```python
from build123d import *

# Parameters (mm, degrees)
F1_DEPTH  = 40
F3_DEPTH  = 15
F4_DEPTH  = 20
F6_DEPTH  = 15
F8_DEPTH  = 15
F9_R      = 7.5
F10_DEPTH = 70
F13_DEPTH = 6
F11_W     = 22
F11_H     = 56
F14_DEPTH = 6
F15_R     = 9.5
F16_DEPTH = 30
F15_R_2   = 19.5
F17_DEPTH = 12
F18_R     = 10


with BuildPart() as f1:
    # F0 (on Front) → F1 (new body, symmetric)
    with BuildSketch(Plane.XZ):
        Polygon((-30.7818128993, 84.5723358707), (0, 0), (130, 0), (130, 15), (115, 15), (45, 15), (10.5031130731, 15), (-11.5561214376, 75.6072487088), (22.2728129107, 87.9199738686), (17.1425107608, 102.0153631803), align=None)
    extrude(amount=F1_DEPTH, both=True)

    # F2 (on face) → F3 (join)
    with BuildSketch(Plane(origin=(-30.7818128993, 0, 84.5723358707), x_dir=(0.9396926208, 0, 0.3420201433), z_dir=(-0.3420201433, 0, 0.9396926208))):
        with BuildLine():
            Line((51, 40), (51, -40))
            ThreePointArc((51, -40), (91, 0), (51, 40))
        make_face()
    extrude(amount=-F3_DEPTH)

    # F0 (on Front) → F4 (join, symmetric)
    with BuildSketch(Plane.XZ):
        Polygon((-30.7818128993, 84.5723358707), (0, 0), (130, 0), (130, 15), (115, 15), (45, 15), (10.5031130731, 15), (-11.5561214376, 75.6072487088), (22.2728129107, 87.9199738686), (17.1425107608, 102.0153631803), align=None)
        Polygon((45, 15), (115, 15), (115, 55), (100, 55), (100, 22), (60, 22), (60, 55), (45, 55), align=None)
    extrude(amount=F4_DEPTH, both=True)

    # F5 (on face) → F6 (join)
    with BuildSketch(Plane.YZ.offset(115)):
        with BuildLine():
            Line((-20, 55), (20, 55))
            ThreePointArc((20, 55), (0, 75), (-20, 55))
        make_face()
    extrude(amount=-F6_DEPTH)

    # F7 (on face) → F8 (join)
    with BuildSketch(Plane.YZ.offset(60)):
        with BuildLine():
            Line((-20, 55), (20, 55))
            ThreePointArc((20, 55), (0, 75), (-20, 55))
        make_face()
    extrude(amount=-F8_DEPTH)

    # F9 (on face) → F10 (cut)
    with BuildSketch(Plane.YZ.offset(115)):
        with Locations((0, 55)):
            Circle(F9_R)
    extrude(amount=-F10_DEPTH, mode=Mode.SUBTRACT)

    # F12 (on face) → F13 (cut)
    with BuildSketch(Plane(origin=(-30.7818128993, 0, 84.5723358707), x_dir=(0.9396926208, 0, 0.3420201433), z_dir=(-0.3420201433, 0, 0.9396926208))):
        with BuildLine():
            Line((89.4577690461, 11), (0, 11))
            Line((0, 11), (0, -11))
            Line((0, -11), (89.4577690461, -11))
            ThreePointArc((89.4577690461, -11), (91, 0), (89.4577690461, 11))
        make_face()
    extrude(amount=-F13_DEPTH, mode=Mode.SUBTRACT)

    # F11 (on face) → F14 (cut)
    with BuildSketch(Plane(origin=(0, 0, 0), x_dir=(0, -1, 0), z_dir=(-0.9396926208, 0, -0.3420201433))):
        with Locations((0, 62)):
            Rectangle(F11_W, F11_H)
    extrude(amount=-F14_DEPTH, mode=Mode.SUBTRACT)

    # F15 (on face) → F16 (cut)
    with BuildSketch(Plane(origin=(-30.7818128993, 0, 84.5723358707), x_dir=(0.9396926208, 0, 0.3420201433), z_dir=(-0.3420201433, 0, 0.9396926208))):
        with Locations((51, 0)):
            Circle(F15_R)
    extrude(amount=-F16_DEPTH, mode=Mode.SUBTRACT)

    # F15 (on face) → F17 (cut)
    with BuildSketch(Plane(origin=(-30.7818128993, 0, 84.5723358707), x_dir=(0.9396926208, 0, 0.3420201433), z_dir=(-0.3420201433, 0, 0.9396926208))):
        with Locations((51, 0)):
            Circle(F15_R_2)
        with Locations((51, 0)):
            Circle(F15_R, mode=Mode.SUBTRACT)
    extrude(amount=-F17_DEPTH, mode=Mode.SUBTRACT)

    # F18
    f18_edges = [f1.edges().sort_by_distance(p)[0] for p in [
        (-11.556121, 0, 75.607249),
        (10.503113, 0, 15),
    ]]
    fillet(f18_edges, radius=F18_R)


solid = f1.part
```
Design review of the part built by this model. Coordinates are the model's own, in mm. A direction names the side the tool comes from. Round coordinates to 2 decimals unless told otherwise and drop trailing zeros. Order: outer loops, then holes, each group sorted by start corner. A loop starts at its lowest first (then second) coordinate and runs counter-clockwise, first axis right, second up. Notation, with made-up numbers: (-9, 45) - (29, 45) arc R8 cw to (29, 56) - close; hole circle Ø2 at (70.5, 52). An arc over 180 degrees is marked (long way). One line per question, with ' | ' between items.
Item 1: Draft analysis for pull direction X (two halves, no side actions). For faces 5 (the face through (44, 11, 109)), 6 (the face through (-8.85, 0.15, 32.96)), 7 (the face through (60, 0, 43)), state which applies: +X half, -X half, draft (parallel to the pull), parting line (faces both ways), or undercut.
Checks:
face 5: draft | face 6: -X half | face 7: undercut
Item 2: Take a section at B-B, the plane y = 31. Write out the cut boundary in (x, z), then the cut area to 3 significant figures.
Checks:
outline: (-30.78, 84.57) - (0, 0) - (130, 0) - (130, 15) - (17.51, 15) arc R10 cw to (8.11, 21.58) - (-8.14, 66.21) arc R10 cw to (-2.16, 79.03) - (46.03, 96.57) - (40.9, 110.66) - close | area: 4,090 mm²
Item 3: Wall thickness on line 1 (Z direction, x = 105, y = 0); line 2 (X direction, y = -1, z = 38.5); line 3 (Z direction, x = 119, y = -24.5): over which ranges is each line inside the solid? List them lowest first. Write a range as [from, to].
Checks:
line 1: [0, 47.5], [62.5, 75] | line 2: [-7.63, 1.95], [45, 60], [100, 115] | line 3: [0, 15]
Item 4: Machinability: for faces 1 (the face through (80, 0, 22)), 2 (the face through (-7.848, -0.56, 73.757)), 3 (the face through (12.846, -4.06, 87.682)), 4 (the face through (115, 0, 45)), which of the approach directions +Z, -Z, +X, -X, +Y, -Y give a long, thin tool a straight path to every point of the face, cutting with its end or side? Answer none if there is none.
Checks:
face 1: +Z, +Y, -Y | face 2: +Y, -Y | face 3: none | face 4: +Z, +X, +Y, -Y
Item 5: For P1, Ø10.5, axis at x = 40, z = 108, coming from the +Y side; P2, Ø6.5, axis at x = 45.5, z = 107.5, coming from the -Y side; P3, Ø20, axis at y = 2, z = 47.5, coming from the +X side; P4, Ø1, axis at x = 2.5, y = 8.5, coming from the -Z side, all flat-tipped, find the tip position at first contact; note any pin that passes through.
Checks:
P1: y = 35.58 | P2: y = -31 | P3: x = 115 | P4: z = 0
Item 6: Take a section at A-A, the plane x = 83.5. Write out the cut boundary in (y, z).
Checks:
outline: (-40, 0) - (40, 0) - (40, 15) - (20, 15) - (20, 22) - (-20, 22) - (-20, 15) - (-40, 15) - close
Item 7: Take a section at C-C, the plane x = 48. Give the number of separate pieces and of enclosed holes in the cut face, then the cut area to 3 significant figures.
Checks:
separate pieces: 2 | enclosed holes: 1 | area: 3,950 mm²
